Source: CAD feature listing. Evaluate the final solid. Frame: model axes, mm. Coordinates: 2 decimals unless noted, no trailing zeros. Loops run counter-clockwise (first coordinate to the right, second up) from the corner with the lowest first, then second, coordinate; pieces in that order, holes last. Notation, with made-up numbers: (31.5, -34) -> (63.5, -34) arc R17 ccw to (63.5, -4) -> close; hole circle Ø7 at (-23, 10). An arc over 180 degrees is marked (long way). Answer as a JSON object with one key per item and string values. Group by question number.
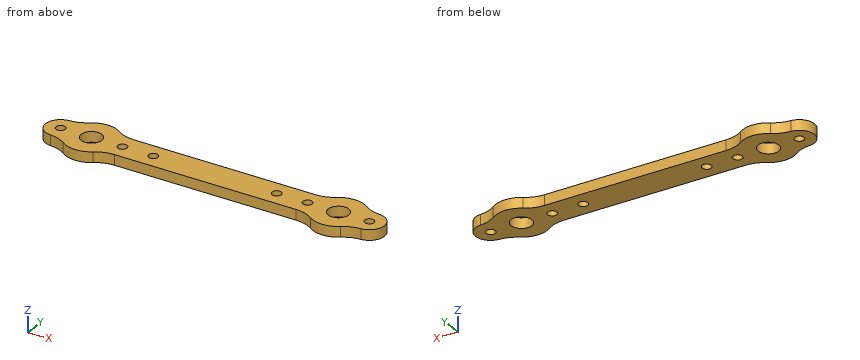
from build123d import *

# Parameters (mm, degrees)
F0_R     = 0.9
F0_R_2   = 2
F1_DEPTH = 2


with BuildPart() as f1:
    # F0 (on Top) → F1 (new body)
    with BuildSketch(Plane.XY):
        with BuildLine():
            Line((17.675445, 3), (0, 3))
            Line((0, 3), (-17.675445, 3))
            ThreePointArc((-17.675445, 3), (-19.484513, 3.279224), (-21.125202, 4.090909))
            ThreePointArc((-21.125202, 4.090909), (-24.044149, 4.999805), (-26.946591, 4.039505))
            ThreePointArc((-26.946591, 4.039505), (-28.468983, 3.234854), (-30.157219, 2.895735))
            ThreePointArc((-30.157219, 2.895735), (-32.9, 0), (-30.157219, -2.895735))
            ThreePointArc((-30.157219, -2.895735), (-28.468983, -3.234854), (-26.946591, -4.039505))
            ThreePointArc((-26.946591, -4.039505), (-24.044149, -4.999805), (-21.125202, -4.090909))
            ThreePointArc((-21.125202, -4.090909), (-19.484513, -3.279224), (-17.675445, -3))
            Line((-17.675445, -3), (0, -3))
            Line((0, -3), (17.675445, -3))
            ThreePointArc((17.675445, -3), (19.484513, -3.279224), (21.125202, -4.090909))
            ThreePointArc((21.125202, -4.090909), (24.044149, -4.999805), (26.946591, -4.039505))
            ThreePointArc((26.946591, -4.039505), (28.468983, -3.234854), (30.157219, -2.895735))
            ThreePointArc((30.157219, -2.895735), (32.9, 0), (30.157219, 2.895735))
            ThreePointArc((30.157219, 2.895735), (28.468983, 3.234854), (26.946591, 4.039505))
            ThreePointArc((26.946591, 4.039505), (24.044149, 4.999805), (21.125202, 4.090909))
            ThreePointArc((21.125202, 4.090909), (19.484513, 3.279224), (17.675445, 3))
        make_face()
        with Locations((-30, 0)):
            Circle(F0_R, mode=Mode.SUBTRACT)
        with Locations((-24, 0)):
            Circle(F0_R_2, mode=Mode.SUBTRACT)
        with Locations((-18, 0)):
            Circle(F0_R, mode=Mode.SUBTRACT)
        with Locations((-12, 0)):
            Circle(F0_R, mode=Mode.SUBTRACT)
        with Locations((12, 0)):
            Circle(F0_R, mode=Mode.SUBTRACT)
        with Locations((18, 0)):
            Circle(F0_R, mode=Mode.SUBTRACT)
        with Locations((24, 0)):
            Circle(F0_R_2, mode=Mode.SUBTRACT)
        with Locations((30, 0)):
            Circle(F0_R, mode=Mode.SUBTRACT)
    extrude(amount=F1_DEPTH)


solid = f1.part
1. Ray query, L1, parallel to Y at x = 12, z = 0.85; L2, parallel to Y at x = -24, z = 0.5; L3, parallel to X at y = 1.25, z = 0.9. Return the intervals inside material, ascending.
2. Section query B-B on z = 0.9. State how many separate pieces and enclosed holes the cut face has, then the cut area to 3 significant figures.
3. Section query C-C on x = 12. Return loops of the section in (y, z).
4. Pin query (flat end, axial travel): pin 1 Ø1.4 at (x, y) = (-12, 0) entering from -Z; pin 2 Ø1 at (x, z) = (-1.5, 1) entering from +Y. Return the tip coordinate at first contact, or that it passes through.
5. Section query A-A on x = -24. Return loops of the section in (y, z), then the cut area to 3 significant figures.
Solved:
{
 "1": {"L1": "-3 to -0.9, 0.9 to 3", "L2": "-5 to -2, 2 to 5", "L3": "-32.62 to -25.56, -22.44 to 22.44, 25.56 to 32.62"},
 "2": {"separate pieces": "1", "enclosed holes": "8", "area": "394 mm^2"},
 "3": {"outline": "(-3, 0) -> (-0.9, 0) -> (-0.9, 2) -> (-3, 2) -> close; (0.9, 0) -> (3, 0) -> (3, 2) -> (0.9, 2) -> close"},
 "4": {"pin 1": "through", "pin 2": "y = 3"},
 "5": {"outline": "(-5, 0) -> (-2, 0) -> (-2, 2) -> (-5, 2) -> close; (2, 0) -> (5, 0) -> (5, 2) -> (2, 2) -> close", "area": "12.0 mm^2"}
}
